from build123d import *

# Parameters (mm, degrees)
SKETCH1_W           = 7
SKETCH1_H           = 6
BOSS_EXTRUDE1_DEPTH = 9
SKETCH2_OUTSIDE_W   = 11.576
SKETCH2_OUTSIDE_H   = 13.576
CUT_EXTRUDE1_DEPTH  = 3
SKETCH3_W           = 3
SKETCH3_H           = 5
CUT_EXTRUDE2_DEPTH  = 1
SKETCH4_W           = 2
SKETCH4_H           = 3
CUT_EXTRUDE3_DEPTH  = 2
CUT_EXTRUDE4_DEPTH  = 2


with BuildPart() as part:
    # Sketch1 → Boss-Extrude1 (new body)
    with BuildSketch(Plane.XY):
        Rectangle(SKETCH1_W, SKETCH1_H)
    extrude(amount=BOSS_EXTRUDE1_DEPTH)

    # Sketch2 outside → Cut-Extrude1 (cut)
    with BuildSketch(Plane(origin=(0, 3, 0), x_dir=(1, 0, 0), z_dir=(0, 1, 0))):
        with Locations((0, -4.5)):
            Rectangle(SKETCH2_OUTSIDE_W, SKETCH2_OUTSIDE_H)
        Polygon((2.5, 0), (2.5, -1), (1.5, -2), (-0.5, -2), (-0.5, -3), (-1.5, -3), (-1.5, -6), (-3.5, -6), (-3.5, 0), align=None, mode=Mode.SUBTRACT)
    extrude(amount=-CUT_EXTRUDE1_DEPTH, mode=Mode.SUBTRACT)

    # Sketch3 → Cut-Extrude2 (cut)
    with BuildSketch(Plane(origin=(0, 0, 0), x_dir=(1, 0, 0), z_dir=(0, 1, 0))):
        with Locations((2, -6.5)):
            Rectangle(SKETCH3_W, SKETCH3_H)
    extrude(amount=-CUT_EXTRUDE2_DEPTH, mode=Mode.SUBTRACT)

    # Sketch4 → Cut-Extrude3 (cut)
    with BuildSketch(Plane(origin=(0, -1, 0), x_dir=(1, 0, 0), z_dir=(0, 1, 0))):
        with Locations((2.5, -7.5)):
            Rectangle(SKETCH4_W, SKETCH4_H)
    extrude(amount=-CUT_EXTRUDE3_DEPTH, mode=Mode.SUBTRACT)

    # Sketch5 → Cut-Extrude4 (cut)
    with BuildSketch(Plane(origin=(-1.5, 0, 0), x_dir=(0, 0, -1), z_dir=(1, 0, 0))):
        Polygon((-4, 3), (-6, 1), (-6, 3), align=None)
    extrude(amount=-CUT_EXTRUDE4_DEPTH, mode=Mode.SUBTRACT)


solid = part.part
Input: part model. Units: mm. Frame: model coordinates. A direction names the side the tool comes from. Give positions to 0.01 mm unless a question says otherwise; leave off trailing zeros. Order: outer loops, then holes, each group sorted by start corner. A loop starts at its lowest first (then second) coordinate and runs counter-clockwise, first axis right, second up. Notation, with made-up numbers: (-32, 14) - (-3, 14) arc R28 cw to (-3, 39) - close; hole circle Ø3 at (-1.5, -12). An arc over 180 degrees is marked (long way). Write each question's results on one line, items separated by ' | '.
Item 1: Contact query for flat-ended pins moving along their axis: pin 1 Ø0.8 at (y, z) = (1, 0.5) entering from +X; pin 2 Ø1.1 at (y, z) = (2, 2.5) entering from +X; pin 3 Ø1.6 at (x, y) = (0.5, 2) entering from +Z. Output: stop coordinate, or through.
A:
pin 1: stops at x = 2.5 | pin 2: stops at x = 1.55 | pin 3: stops at z = 2
Item 2: Section D-D (x = 1.75). Return loops of the section in (y, z), and give its area (4 significant figures).
A:
outline: (-3, 0) - (3, 0) - (3, 1.75) - (0, 1.75) - (0, 4) - (-1, 4) - (-1, 6) - (-3, 6) - close | area: 21.25 mm^2
Item 3: Section C-C (z = 0.5). Return loops of the section in (x, y), and give its area (3 significant figures).
A:
outline: (-3.5, -3) - (3.5, -3) - (3.5, 0) - (2.5, 0) - (2.5, 3) - (-3.5, 3) - close | area: 39.0 mm^2
Item 4: Section B-B (y = 1.6). Return loops of the section in (x, z).
A:
outline: (-3.5, 0) - (2.5, 0) - (2.5, 1) - (1.5, 2) - (-0.5, 2) - (-0.5, 3) - (-1.5, 3) - (-1.5, 5.4) - (-3.5, 5.4) - close
Item 5: Access query for faces 1 (the flat face through (1.5, -2, 8)), 2 (the flat face through (-1.5, 1, 4)), 3 (the flat face through (2.5, 1.5, 0.5)). Directions: +Z, -Z, +X, -X, +Y, -Y. A direction counts if a zero-diameter tool reaches every point of the face in a straight line with its end or side. Return the directions, or none.
A:
face 1: +Z, +X, +Y, -Y | face 2: +Z, +X, +Y | face 3: +Z, -Z, +X, +Y
Item 6: Material intervals for line 1 along Z through (x, y) = (3, -1.85); line 2 along Y through (x, z) = (-1.5, 7.75); line 3 along X through (y, z) = (0.2, 4.5), sorted ascending.
A:
line 1: z = 0 to 6 | line 2: y = -3 to 0 | line 3: x = -3.5 to -1.5
Item 7: Section A-A (x = 1). Return loops of the section in (y, z).
A:
outline: (-3, 0) - (3, 0) - (3, 2) - (0, 2) - (0, 4) - (-1, 4) - (-1, 9) - (-3, 9) - close
